Answer from the drawing. Dimensions are ordinates in mm from the lowest x, y and z of the part. Coordinates: 2 decimals unless noted, no trailing zeros. Loops run counter-clockwise (first coordinate to the right, second up) from the corner with the lowest first, then second, coordinate; pieces in that order, holes last.
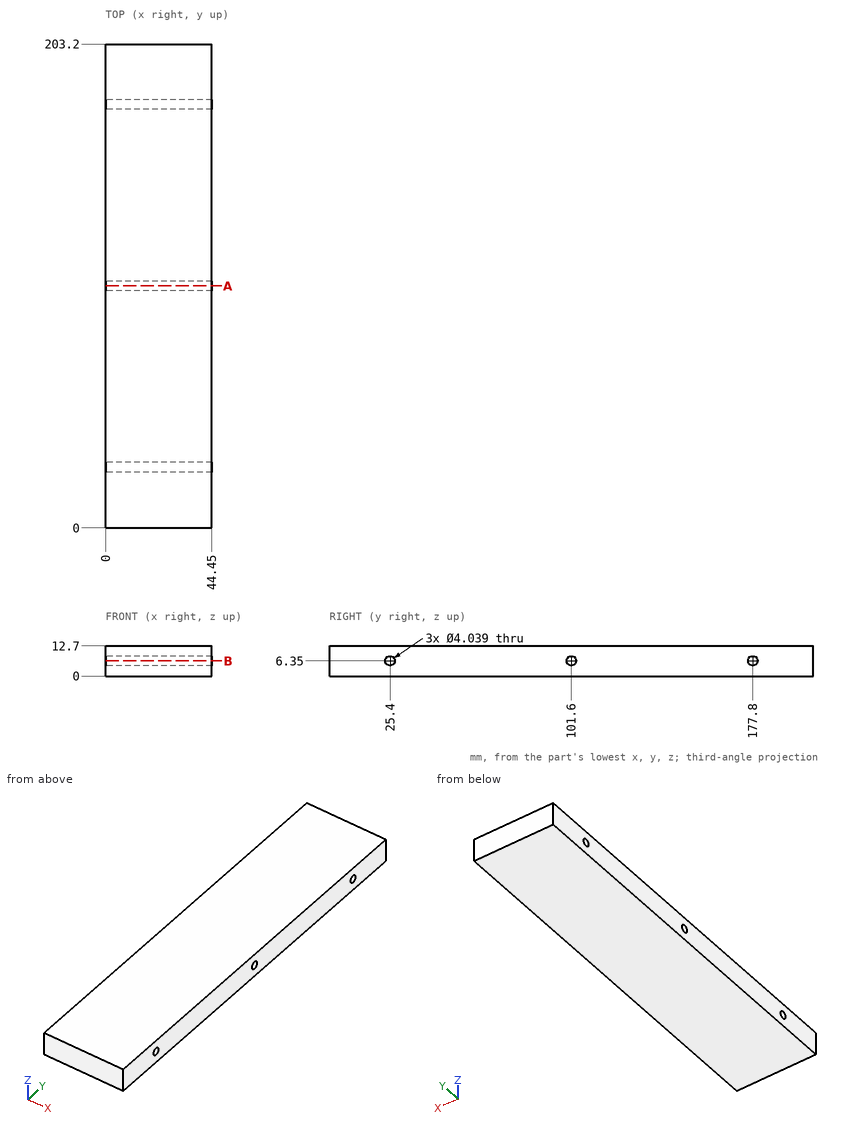
Item 1: A cutting plane is placed at A-A on y = 101.6. Determine the outline of the cut face in (x, z), then the cut area to 3 significant figures.
Numbers:
outline: (0, 0) - (44.45, 0) - (44.45, 4.33) - (0, 4.33) - close; (0, 8.37) - (44.45, 8.37) - (44.45, 12.7) - (0, 12.7) - close
area: 385 mm2
Item 2: A cutting plane is placed at B-B on z = 6.35. Determine the outline of the cut face in (x, y), then the cut area to 3 significant figures.
Numbers:
outline: (0, 0) - (44.45, 0) - (44.45, 23.38) - (0, 23.38) - close; (0, 27.42) - (44.45, 27.42) - (44.45, 99.58) - (0, 99.58) - close; (0, 103.62) - (44.45, 103.62) - (44.45, 175.78) - (0, 175.78) - close; (0, 179.82) - (44.45, 179.82) - (44.45, 203.2) - (0, 203.2) - close
area: 8,490 mm2
Item 3: Find the intervals of material crossed by line 1 along Y through (x, z) = (30.5, 6.35); line 2 along Z through (x, y) = (17, 25); line 3 along Z through (x, y) = (14, 177.8), in increasing order.
Numbers:
line 1: y = 0 to 23.38, 27.42 to 99.58, 103.62 to 175.78, 179.82 to 203.2
line 2: z = 0 to 4.37, 8.33 to 12.7
line 3: z = 0 to 4.33, 8.37 to 12.7
